```python
from build123d import *

# Parameters (mm, degrees)
SKETCH1_W           = 254
SKETCH1_H           = 43
BOSS_EXTRUDE1_DEPTH = 0.2
BOSS_EXTRUDE2_DEPTH = 254


with BuildPart() as part:
    # Sketch1 → Boss-Extrude1 (new body)
    with BuildSketch(Plane(origin=(0, 0, 0), x_dir=(1, 0, 0), z_dir=(0, 1, 0))):
        with Locations((-6.018162295, 0)):
            Rectangle(SKETCH1_W, SKETCH1_H)
    extrude(amount=BOSS_EXTRUDE1_DEPTH)

    # Sketch4 → Boss-Extrude2 (add)
    with BuildSketch(Plane(origin=(-133.018162295, 0, 0), x_dir=(0, 0, -1), z_dir=(1, 0, 0))):
        with BuildLine():
            Line((21.5, 0.2), (21.5, 3.005611905))
            ThreePointArc((21.5, 3.005611905), (22.439298034, 3.944909939), (21.5, 4.884207973))
            Line((21.5, 4.884207973), (21.5, 9.2))
            Line((21.5, 9.2), (21.317120226, 9.402181424))
            add(Edge.make_bspline(
                [(21.317120226, 9.402181424), (19.631812119, 9.571563167), (17.951135022, 9.796064061), (16.280476178, 10.075084883)],
                knots=[0, 0, 0, 0, 1, 1, 1, 1], degree=3))
            Line((16.280476178, 10.075084883), (16.247002876, 9.874660887))
            add(Edge.make_bspline(
                [(21.2968, 9.2), (18.759973351, 9.454963539), (16.247002876, 9.874660887)],
                knots=[0, 0, 0, 1, 1, 1], degree=2))
            Line((21.2968, 9.2), (21.2968, 4.652405576))
            ThreePointArc((21.2968, 4.652405576), (22.236098034, 3.944909939), (21.2968, 3.237414303))
            Line((21.2968, 3.237414303), (21.2968, 0.2))
            Line((21.2968, 0.2), (21.5, 0.2))
        make_face()
    boss_extrude2 = extrude(amount=BOSS_EXTRUDE2_DEPTH)

    # Mirror1: Boss-Extrude2 across plane
    add(boss_extrude2.mirror(Plane.XY))


solid = part.part
```
Check sheet for the modelled part. Datum: model origin and axes. Units: mm. A direction names the side the tool comes from. Coordinates: 2 decimals unless noted, no trailing zeros. Order: outer loops, then holes, each group sorted by start corner. A loop starts at its lowest first (then second) coordinate and runs counter-clockwise, first axis right, second up. Notation, with made-up numbers: M 0.5,89.5 L 37.5,89.5 A19 ccw 37.5,95.5 Z; hole C 5,-27.75 d7. An arc over 180 degrees is marked long. Write each question's results on one line, items separated by ' | '. Start each with the question number.
1. Cross-section at A-A on y = 6.75. Record the cut outline in (x, z), and give its area (3 significant figures).
2. Cross-section at B-B on z = -13. Record the cut outline in (x, y).
3. Mould release check, pull along Y, two halves, no side actions. Record for faces 3 (the face through (-8, 7, -21.297)), 4 (the face through (-8, 7, 21.5)), 5 (the face through (-8, 0, 0)): +Y half, -Y half, draft (parallel to the pull), parting line (faces both ways), or undercut.
4. Go/stop test with flat-tipped pins: P1, Ø1.3, axis at x = -63.5, y = 6, coming from the +Z side; P2, Ø2.5, axis at x = 10, y = 1, coming from the -Z side; P3, Ø1, axis at x = 35, z = -6.5, coming from the +Y side; P4, Ø2, axis at y = 1.5, z = -4, coming from the +X side. Record where each tip stops, or that it passes through.
5. Material ranges on probe 1 along Z at (x, y) = (-62, 8.5); probe 2 along Y at (x, z) = (-72, 21); probe 3 along Y at (x, z) = (-88, 17.5), recorded low to high.
6. Access from +Z, -Z, +X, -X, +Y, -Y to the whole of each face (thin tool, end or side, straight path). Record for faces 1 (the face through (-8, 0.2, 0)), 2 (the face through (-8, 7, -21.5)).
Checks:
1) outline: M -133.02,-21.5 L 120.98,-21.5 L 120.98,-21.3 L -133.02,-21.3 Z; M -133.02,21.3 L 120.98,21.3 L 120.98,21.5 L -133.02,21.5 Z | area: 103 mm²
2) outline: M -133.02,0 L 120.98,0 L 120.98,0.2 L -133.02,0.2 Z
3) face 3: undercut | face 4: draft | face 5: -Y half
4) P1: stops at z = 21.5 | P2: stops at z = -21.5 | P3: stops at y = 0.2 | P4: passes through
5) probe 1: z = -21.5 to -21.3, 21.3 to 21.5 | probe 2: y = 0 to 0.2, 9.23 to 9.43 | probe 3: y = 0 to 0.2, 9.68 to 9.88
6) face 1: +X, -X | face 2: -Z, +X, -X, +Y
